Could you check a few things on this model? Use its own coordinates, in mm. Face numbers are marked on the shaded views. A direction names the side the tool comes from. Round coordinates to 2 decimals unless told otherwise and drop trailing zeros. Loops run counter-clockwise (first coordinate to the right, second up) from the corner with the lowest first, then second, coordinate; pieces in that order, holes last. Notation, with made-up numbers: M -19,15.25 L 20,15.25 A14 ccw 20,26.25 Z; hole C 11,-5.5 d1. An arc over 180 degrees is marked long. Return JSON: item names as keys, results as strings. Group by question number.
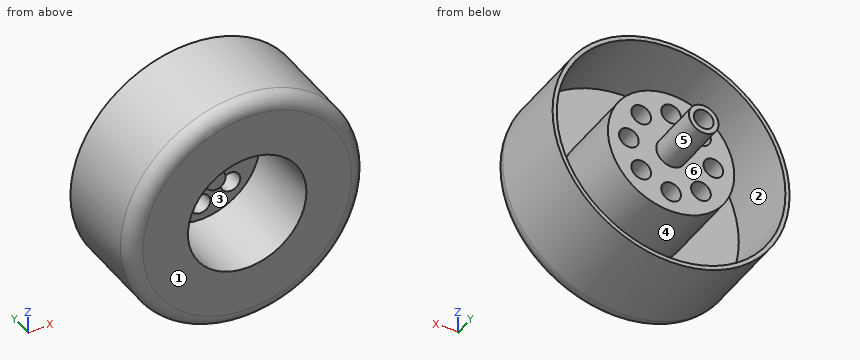
```python
from build123d import *

# Parameters (mm, degrees)
F0_R      = 19.05
F1_DEPTH  = 15.875
F2_R      = 9.525
F3_DEPTH  = 12.7
F4_R      = 18.3769
F4_R_2    = 10.16
F5_DEPTH  = 12.7
F6_R      = 1.5875
F7_DEPTH  = 25.4
F8_R      = 3.175
F9_DEPTH  = 1.5875
F10_R     = 1.5875
F11_DEPTH = 2.54
F12_R     = 0.254
F13_DEPTH = 0.508
F14_R     = 2.38125
F14_R_2   = 1.5875
F15_DEPTH = 8.89
F16_R     = 2.286


with BuildPart() as f1:
    # F0 (on Front) → F1 (new body)
    with BuildSketch(Plane.XZ):
        Circle(F0_R)
    extrude(amount=F1_DEPTH)

    # F2 (on face) → F3 (cut)
    with BuildSketch(Plane.XZ.offset(15.875)):
        Circle(F2_R)
    extrude(amount=-F3_DEPTH, mode=Mode.SUBTRACT)

    # F4 (on face) → F5 (cut)
    with BuildSketch(Plane(origin=(0, 0, 0), x_dir=(-1, 0, 0), z_dir=(0, 1, 0))):
        Circle(F4_R)
        Circle(F4_R_2, mode=Mode.SUBTRACT)
    extrude(amount=-F5_DEPTH, mode=Mode.SUBTRACT)

    # F6 (on face) → F7 (cut)
    with BuildSketch(Plane.XZ.offset(3.175)):
        with BuildLine():
            ThreePointArc((0, 5.2043736776), (1.1225320151, 5.6693416624), (1.5875, 6.7918736776))
            ThreePointArc((1.5875, 6.7918736776), (-1.1225320151, 7.9144056927), (0, 5.2043736776))
        make_face()
        with Locations((-4.8025799344, 4.8025799344)):
            Circle(F6_R)
        with Locations((-6.7918736776, 0)):
            Circle(F6_R)
        with Locations((-4.8025799344, -4.8025799344)):
            Circle(F6_R)
        with Locations((0, -6.7918736776)):
            Circle(F6_R)
        with Locations((4.8025799344, -4.8025799344)):
            Circle(F6_R)
        with Locations((6.7918736776, 0)):
            Circle(F6_R)
        with Locations((4.8025799344, 4.8025799344)):
            Circle(F6_R)
    extrude(amount=-F7_DEPTH, mode=Mode.SUBTRACT)

    # F8 (on face) → F9 (join)
    with BuildSketch(Plane.XZ.offset(3.175)):
        Circle(F8_R)
    extrude(amount=F9_DEPTH)

    # F10 (on face) → F11 (join)
    with BuildSketch(Plane.XZ.offset(4.7625)):
        Circle(F10_R)
    extrude(amount=F11_DEPTH)

    # F12 (on face) → F13 (join)
    with BuildSketch(Plane.XZ.offset(4.7625)):
        with BuildLine():
            ThreePointArc((0, 2.6449868941), (-0.254, 2.3909868941), (0, 2.1369868941))
            Line((0, 2.1369868941), (0, 2.6449868941))
        make_face()
        with BuildLine():
            Line((0, 2.6449868941), (0, 2.1369868941))
            ThreePointArc((0, 2.1369868941), (0.1796051224, 2.2113817717), (0.254, 2.3909868941))
            ThreePointArc((0.254, 2.3909868941), (0.1796051224, 2.5705920165), (0, 2.6449868941))
        make_face()
        with Locations((1.4053868348, 1.9343490307)):
            Circle(F12_R)
        with Locations((2.273963666, 0.7388555836)):
            Circle(F12_R)
        with Locations((2.273963666, -0.7388555836)):
            Circle(F12_R)
        with Locations((0, -2.3909868941)):
            Circle(F12_R)
        with Locations((-1.4053868348, -1.9343490307)):
            Circle(F12_R)
        with Locations((1.4053868348, -1.9343490307)):
            Circle(F12_R)
        with Locations((-2.273963666, 0.7388555836)):
            Circle(F12_R)
        with Locations((-1.4053868348, 1.9343490307)):
            Circle(F12_R)
        with Locations((-2.273963666, -0.7388555836)):
            Circle(F12_R)
    extrude(amount=F13_DEPTH)

    # F14 (on face) → F15 (join)
    with BuildSketch(Plane(origin=(0, 0, 0), x_dir=(-1, 0, 0), z_dir=(0, 1, 0))):
        Circle(F14_R)
        Circle(F14_R_2, mode=Mode.SUBTRACT)
    extrude(amount=F15_DEPTH)

    # F16
    f16_edges = [f1.edges().sort_by_distance(p)[0] for p in [
        (-19.05, -15.875, 0),
    ]]
    fillet(f16_edges, radius=F16_R)


solid = f1.part
```
1. We'd pull the mould along X, two halves only. Please class the marked faces 4, 5 and 6: +X half, -X half, draft (parallel to the pull), parting line (faces both ways), or undercut.
2. If we section it at A-A, the plane y = -11.25: Please give me the cut outline in (x, z) (3 decimals), then the cut area to 3 significant figures.
3. I need wall thicknesses on probe 1 along Z at (x, y) = (0, -0.95); probe 2 along X at (y, z) = (-8.25, -2); probe 3 along Z at (x, y) = (8, -5). Which ranges of each line are inside material? Lowest first, please.
4. I'm going to push flat-ended pins straight in: pin 1 Ø8 at (y, z) = (6, -8.5) entering from -X; pin 2 Ø10 at (x, y) = (7.5, -13.5) entering from -Z; pin 3 Ø1 at (x, z) = (-11.5, 4.5) entering from +Y; pin 4 Ø6 at (x, y) = (2, -2) entering from +Z. Where does each tip first touch, or does it pass through?
5. If we section it at B-B, the plane z = 0: Give the number of separate pieces and of enclosed holes in the cut face, then the cut area to 3 significant figures.
6. On a 3-axis mill with a long thin cutter (end or side, diameter ignored), from which of +Z, -Z, +X, -X, +Y, -Y can I reach the whole of each face in a straight line? I mean the marked faces 1, 2 and 3. Say none if no direction works.
Geometry results:
{
 "1": {"face 4": "undercut", "face 5": "parting line", "face 6": "draft"},
 "2": {"outline": "C 0,0 d38.1; C 0,0 d20.32; hole C 0,0 d36.754; hole C 0,0 d19.05", "area": "118 mm^2"},
 "3": {"probe 1": "-19.05 to -18.38, -10.16 to -8.38, -5.2 to 5.2, 8.38 to 10.16, 18.38 to 19.05", "probe 2": "-18.94 to -18.27, -9.96 to -9.31, 9.31 to 9.96, 18.27 to 18.94", "probe 3": "-17.29 to -16.54, -6.26 to -5.17, 5.17 to 6.26, 16.54 to 17.29"},
 "4": {"pin 1": "through", "pin 2": "z = -18.89", "pin 3": "y = -12.7", "pin 4": "z = 19.05"},
 "5": {"separate pieces": "3", "enclosed holes": "0", "area": "164 mm^2"},
 "6": {"face 1": "+Z, -Z, +X, -X, -Y", "face 2": "+Y", "face 3": "-Y"}
}
